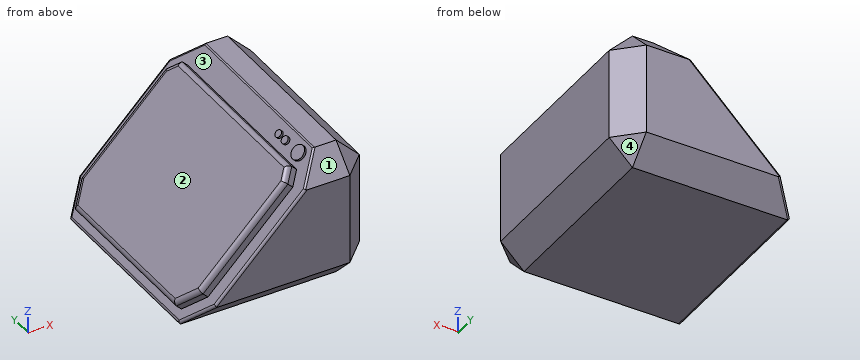
from build123d import *

# Parameters (mm, degrees)
F1_DEPTH = 50
F3_DEPTH = 2.5
F4_R     = 1
F5_R     = 1.6151714505
F5_R_2   = 0.8396882265
F5_R_3   = 0.796597451
F6_DEPTH = 0.5
F7_SIZE  = 5.08
F8_R     = 0.5


with BuildPart() as f1:
    # F0 (on Front) → F1 (new body)
    with BuildSketch(Plane.XZ):
        Polygon((3.6212546234, 51.0512575135), (-26.3787453766, 21.0512575135), (13.6212546234, 21.0512575135), (13.6212546234, 51.0512575135), align=None)
    extrude(amount=F1_DEPTH)

    # F2 (on face) → F3 (join)
    with BuildSketch(Plane(origin=(-23.715001445, 0, 23.715001445), x_dir=(0.7071067812, 0, 0.7071067812), z_dir=(-0.7071067812, 0, 0.7071067812))):
        Polygon((30.521587444, -47), (33.4631516538, -44.92), (33.4631516538, -5.08), (30.521587444, -3), (4.3706138377, -3), (-0.7671027947, -6.6329142706), (-0.7671027947, -43.3670857294), (4.3706138377, -47), align=None)
    extrude(amount=F3_DEPTH)

    # F4
    f4_edges = [f1.edges().sort_by_distance(p)[0] for p in [
        (-13.146512, -3, 37.819024),
        (-2.860747, -45.96, 48.10479),
        (-1.820747, -25, 49.14479),
        (-2.860747, -4.04, 48.10479),
        (-24.208735, -4.816457, 26.756802),
        (-26.025192, -25, 24.940345),
        (-24.208735, -45.183543, 26.756802),
        (-13.146512, -47, 37.819024),
    ]]
    fillet(f4_edges, radius=F4_R)

    # F5 (on face) → F6 (join)
    with BuildSketch(Plane(origin=(-23.715001445, 0, 23.715001445), x_dir=(0.7071067812, 0, 0.7071067812), z_dir=(-0.7071067812, 0, 0.7071067812))):
        with Locations((36.0333621502, -42.8570471704)):
            Circle(F5_R)
        with Locations((36.0333621502, -38.0774661899)):
            Circle(F5_R_2)
        with Locations((36.0272766753, -35.6876738369)):
            Circle(F5_R_3)
    extrude(amount=F6_DEPTH)

    # F7
    f7_edges = [f1.edges().sort_by_distance(p)[0] for p in [
        (-6.378745, 0, 21.051258),
        (-6.378745, -50, 21.051258),
        (8.621255, -50, 51.051258),
        (13.621255, -50, 36.051258),
        (13.621255, -25, 51.051258),
        (8.621255, 0, 51.051258),
        (13.621255, 0, 36.051258),
        (13.621255, -25, 21.051258),
    ]]
    chamfer(f7_edges, length=F7_SIZE)

    # F8
    f8_edges = [f1.edges().sort_by_distance(p)[0] for p in [
        (-26.378745, -25, 21.051258),
        (-23.838745, -2.54, 23.591258),
        (-11.378745, 0, 36.051258),
        (-23.838745, -47.46, 23.591258),
        (-11.378745, -50, 36.051258),
        (1.081255, -47.46, 48.511258),
        (3.621255, -25, 51.051258),
        (1.081255, -2.54, 48.511258),
    ]]
    fillet(f8_edges, radius=F8_R)


solid = f1.part
Here's how the part is built. I have some questions about the finished solid (model axes, mm). Face numbers are marked on the shaded views. Coordinates: 2 decimals unless noted, no trailing zeros. Write each loop counter-clockwise with the first axis right and the second up, starting at its lowest first coordinate (ties: lowest second). Pieces come first, ordered by that corner, then holes. Notation, with made-up numbers: (-27, -21) - (25, -21) arc R30 cw to (25, 18) - close; hole circle Ø8 at (84.25, -13.5). An arc over 180 degrees is marked (long way). Use one line per item in the form item = value.
1) Suppose I cut it at A-A, the plane y = -26. Write out the boundary of the cut face in (x, z).
Solved:
outline = (-25.53, 21.9) arc R0.5 ccw to (-25.17, 21.05) - (8.54, 21.05) - (13.62, 26.13) - (13.62, 45.97) - (8.54, 51.05) - (3.83, 51.05) arc R0.5 ccw to (3.47, 50.9) - (-0.05, 47.38) - (-1.11, 48.44) arc R1 ccw to (-2.53, 48.44) - (-25.32, 25.65) arc R1 ccw to (-25.32, 24.23) - (-24.26, 23.17) - close
2) I need wall thicknesses on line 1 (Y direction, x = -11, z = 37); line 2 (Z direction, x = -2, y = -45.5); line 3 (Z direction, x = -5, y = -14). Which ranges of each line are inside material? Lowest first, please.
Solved:
line_1 = -47 to -3
line_2 = 21.63 to 48.02
line_3 = 21.05 to 45.97
3) I'm going to push flat-ended pins straight in: P1, Ø5, axis at x = -20, y = -31.5, coming from the +Z side; P2, Ø1, axis at y = -36.5, z = 31.5, coming from the -X side; P3, Ø3, axis at y = -27.5, z = 45, coming from the -X side. Where does each tip first touch, or does it pass through?
Solved:
P1 = 33.47
P2 = -19.97
P3 = -7.47
4) Thinking about a two-plate mould opening in X: for the marked faces 1, 2, 3 and 4, which applies, released by +X, released by -X, zero draft, split by the parting line, or undercut?
Solved:
face_1 = zero draft
face_2 = released by -X
face_3 = undercut
face_4 = released by +X
